CAD build for the part. Positions are in the model's coordinates, mm. A direction names the side the tool comes from. Coordinates: 2 decimals unless noted, no trailing zeros. Order: outer loops, then holes, each group sorted by start corner. A loop starts at its lowest first (then second) coordinate and runs counter-clockwise, first axis right, second up. Notation, with made-up numbers: (32, 71) - (59, 71) arc R30 ccw to (59, 100) - close; hole circle Ø6 at (20, -33.75). An arc over 180 degrees is marked (long way). Use one line per item in the form item = value.
```python
from build123d import *

# Parameters (mm, degrees)
BOSS_EXTRUDE1_DEPTH = 1.5875


with BuildPart() as part:
    # Sketch2 → Boss-Extrude1 (new, symmetric)
    with BuildSketch(Plane.XY):
        with BuildLine():
            Line((0.022257802, 9.82186659), (-2.479270797, 28.706909737))
            Line((-2.479270797, 28.706909737), (-0.263425734, 29.000422426))
            Line((-0.263425734, 29.000422426), (-2.197941184, 43.604855793))
            Line((-2.197941184, 43.604855793), (1.881228135, 44.14518597))
            Line((1.881228135, 44.14518597), (1.547690989, 46.663191723))
            Line((1.547690989, 46.663191723), (-4.747323394, 45.829348857))
            Line((-4.747323394, 45.829348857), (-4.980799396, 47.591952884))
            Line((-4.980799396, 47.591952884), (-15.304622983, 46.224450583))
            Line((-15.304622983, 46.224450583), (-8.733941196, -3.38026275))
            ThreePointArc((-8.733941196, -3.38026275), (-5.154398694, -9.589912307), (1.762103428, -11.470037447))
            Line((1.762103428, -11.470037447), (46.530195884, -5.807878402))
            ThreePointArc((46.530195884, -5.807878402), (52.07, 0.997941592), (45.533364229, 6.85294016))
            Line((45.533364229, 6.85294016), (5.015377017, 5.582956452))
            ThreePointArc((5.015377017, 5.582956452), (1.702583701, 6.740949239), (0.022257802, 9.82186659))
        make_face()
    extrude(amount=BOSS_EXTRUDE1_DEPTH, both=True)


solid = part.part
```
Item 1: 3-axis set-ups, long thin cutter, end or side, ignore diameter. For faces 5 (the face through (-4.862, 46.698, 0.022)), 6 (the face through (23.83, -8.68, 0.02)), 7 (the face through (-0.19, 43.87, 0.02)): which of +Z, -Z, +X, -X, +Y, -Y reach the whole face in a straight line?
Derived:
face_5 = +Z, -Z, +Y
face_6 = +Z, -Z, +X, -Y
face_7 = +Z, -Z, +X
Item 2: Cut at B-B, the plane y = 8.5. Write the cut outline in (x, z), plus the area to 3 significant figures.
Derived:
outline = (-10.31, -1.59) - (0.39, -1.59) - (0.39, 1.59) - (-10.31, 1.59) - close
area = 34.0 mm²
Item 3: Cut at C-C, the plane x = 47.5. Write the cut outline in (y, z), plus the area to 3 significant figures.
Derived:
outline = (-5.61, -1.59) - (6.61, -1.59) - (6.61, 1.59) - (-5.61, 1.59) - close
area = 38.8 mm²
Item 4: Two-plate mould, pull along Y, no slides. Class faces 1 (the face through (10, 5, 1.588)), 2 (the face through (-12.065, 21.769, 0.022)), 3 (the face through (-1.21, 19.13, 0.02)), 4 (the face through (1.74, 6.71, 0.02)): +Y half, -Y half, draft (parallel to the pull), parting line (faces both ways), or undercut.
Derived:
face_1 = draft
face_2 = -Y half
face_3 = undercut
face_4 = undercut
Item 5: Cut at A-A, the plane z = 0.1. Write the cut outline in (x, y).
Derived:
outline = (-15.3, 46.22) - (-8.73, -3.38) arc R9.4 ccw to (1.76, -11.47) - (46.53, -5.81) arc R6.36 ccw to (45.53, 6.85) - (5.02, 5.58) arc R4.88 cw to (0.02, 9.82) - (-2.48, 28.71) - (-0.26, 29) - (-2.2, 43.6) - (1.88, 44.15) - (1.55, 46.66) - (-4.75, 45.83) - (-4.98, 47.59) - close
Item 6: Drill centre lines: line 1 (Y direction, x = 42, z = 0.75); line 2 (X direction, y = 18.5, z = 1); line 3 (X direction, y = 35.5, z = 0.9). Where is each one in solid material? Low to high. Write a range as [from, to].
Derived:
line_1 = [-6.38, 6.74]
line_2 = [-11.63, -1.13]
line_3 = [-13.88, -1.12]
Item 7: Drop flat-ended pins along their axis: pin 1 (1.5 mm diameter, centred on x = 34, z = 0.5, fed in from -Y); pin 2 (1 mm diameter, centred on x = 6.5, z = -1, fed in from +Y); pin 3 (3 mm diameter, centred on x = -0.5, y = 21, fed in from +Z). Give the stop position or say it passes through.
Derived:
pin_1 = -7.49
pin_2 = 5.65
pin_3 = 1.59
